from build123d import *

# Parameters (mm, degrees)
F0_R     = 12.5
F0_R_2   = 3
F1_DEPTH = 56
F0_R_3   = 15.5
F2_DEPTH = 44
F0_R_4   = 28
F3_DEPTH = 40


with BuildPart() as f1:
    # F0 (on Front) → F1 (new body)
    with BuildSketch(Plane.XZ):
        Circle(F0_R)
        Circle(F0_R_2, mode=Mode.SUBTRACT)
    extrude(amount=F1_DEPTH)

    # F0 (on Front) → F2 (join)
    with BuildSketch(Plane.XZ):
        Circle(F0_R_3)
        Circle(F0_R, mode=Mode.SUBTRACT)
    extrude(amount=F2_DEPTH)

    # F0 (on Front) → F3 (join)
    with BuildSketch(Plane.XZ):
        Circle(F0_R_4)
        Circle(F0_R_3, mode=Mode.SUBTRACT)
    extrude(amount=F3_DEPTH)


solid = f1.part
Model file for the job. Use its own axes, mm. A direction names the side the tool comes from. Give positions to 0.01 mm unless a question says otherwise; leave off trailing zeros. Order: outer loops, then holes, each group sorted by start corner. A loop starts at its lowest first (then second) coordinate and runs counter-clockwise, first axis right, second up. Notation, with made-up numbers: M 9.5,-29.5 L 45.5,-29.5 A24 cw 45.5,-9.5 Z; hole C -8.75,47.25 d5. An arc over 180 degrees is marked long. Write item = value, one per line.
Q1. Cut at C-C, the plane y = -8. List the corners of the cut face in (x, z).
Derived:
outline = C 0,0 d56; hole C 0,0 d6
Q2. Tool access for faces 1 (the cylindrical face through (11.923, -49.916, 3.755)), 2 (the cylindrical face through (25.865, -19.72, -10.724)): list every direction of +Z, -Z, +X, -X, +Y, -Y with a clear straight run to the whole face (end or side of a thin tool).
Derived:
face_1 = -Y
face_2 = +Y, -Y
Q3. Cut at A-A, the plane x = 0. List the corners of the cut face in (y, z).
Derived:
outline = M -56,-12.5 L -44,-12.5 L -44,-15.5 L -40,-15.5 L -40,-28 L 0,-28 L 0,-3 L -56,-3 Z; M -56,3 L 0,3 L 0,28 L -40,28 L -40,15.5 L -44,15.5 L -44,12.5 L -56,12.5 Z
Q4. Cut at B-B, the plane z = 0. List the corners of the cut face in (x, y).
Derived:
outline = M -28,-40 L -15.5,-40 L -15.5,-44 L -12.5,-44 L -12.5,-56 L -3,-56 L -3,0 L -28,0 Z; M 3,-56 L 12.5,-56 L 12.5,-44 L 15.5,-44 L 15.5,-40 L 28,-40 L 28,0 L 3,0 Z
Q5. Two-plate mould, pull along Z, no slides. Class faces 3 (the cylindrical face through (-2.018, -41.972, 15.368)), 4 (the flat face through (3, -56, -3)), 5 (the cylindrical face through (-3, -28, 0)): pulls with the +Z half, pulls with the -Z half, needs draft (parallel to the pull), parting line crosses it, or undercut.
Derived:
face_3 = parting line crosses it
face_4 = needs draft
face_5 = undercut
Q6. Cut at D-D, the plane x = -7.5. List the corners of the cut face in (y, z).
Derived:
outline = M -56,-10 L -44,-10 L -44,-13.56 L -40,-13.56 L -40,-26.98 L 0,-26.98 L 0,26.98 L -40,26.98 L -40,13.56 L -44,13.56 L -44,10 L -56,10 Z
Q7. Drill centre lines: line 1 (Z direction, x = 0, y = -36); line 2 (Y direction, x = 22.5, z = -16); line 3 (Y direction, x = 13.5, z = -6.5). Where is each one in solid material? Low to high. Write a range as [from, to].
Derived:
line_1 = [-28, -3], [3, 28]
line_2 = [-40, 0]
line_3 = [-44, 0]
Q8. Flat gauge pins, fed straight in: pin 1 (2 mm diameter, centred on x = -14.5, y = -37.5, fed in from +Z); pin 2 (12 mm diameter, centred on x = -11.5, y = -49, fed in from +Z); pin 3 (6 mm diameter, centred on y = -35, z = -21, fed in from -X). Where does each tip first touch, or does it go through?
Derived:
pin_1 = 24.53
pin_2 = 13.16
pin_3 = -21.45
